Model file for the job. Use its own axes, mm. A direction names the side the tool comes from. Coordinates: 2 decimals unless noted, no trailing zeros. Loops run counter-clockwise (first coordinate to the right, second up) from the corner with the lowest first, then second, coordinate; pieces in that order, holes last.
from build123d import *

# Parameters (mm, degrees)
EXTRUDE_1_DEPTH        = 3.5
EXTRUDE_2_DEPTH        = 1.5
SKETCH_3_OUTSIDE_W     = 10.094
SKETCH_3_OUTSIDE_H     = 10.094
SKETCH_3_OUTSIDE_R     = 2.29
CUT_EXTRUDE_1_DEPTH    = 0.1
SKETCH_4_W             = 1
SKETCH_4_H             = 1.4
EXTRUDE_3_DEPTH        = 0.275
FILLET_1_R             = 0.1
FILLET_1_OF_MIRROR_1_R = 0.1
CUT_EXTRUDE_2_DEPTH    = 2


with BuildPart() as part:
    # 草图1 → 凸台-拉伸1 (new body)
    with BuildSketch(Plane.XY):
        Polygon((-1.91862915, -3.05), (1.91862915, -3.05), (3.05, -1.91862915), (3.05, 1.91862915), (1.91862915, 3.05), (-1.91862915, 3.05), (-3.05, 1.91862915), (-3.05, -1.91862915), align=None)
    extrude(amount=EXTRUDE_1_DEPTH)

    # 草图2 → 凸台-拉伸2 (add)
    with BuildSketch(Plane.XY.offset(3.5)):
        Polygon((2.29, -1.936446609), (1.936446609, -2.29), (-1.936446609, -2.29), (-2.29, -1.936446609), (-2.29, 1.936446609), (-1.936446609, 2.29), (1.936446609, 2.29), (2.29, 1.936446609), align=None)
    extrude(amount=EXTRUDE_2_DEPTH)

    # 草图3 outside → 切除-拉伸1 (cut)
    with BuildSketch(Plane.XY.offset(5)):
        Rectangle(SKETCH_3_OUTSIDE_W, SKETCH_3_OUTSIDE_H)
        Circle(SKETCH_3_OUTSIDE_R, mode=Mode.SUBTRACT)
    cut_extrude_1 = extrude(amount=-CUT_EXTRUDE_1_DEPTH, mode=Mode.SUBTRACT)

    # 草图4 → 凸台-拉伸3 (add)
    with BuildSketch(Plane.ZY.offset(3.05)):
        with Locations((0.5, 0)):
            Rectangle(SKETCH_4_W, SKETCH_4_H)
    extrude_3 = extrude(amount=EXTRUDE_3_DEPTH)

    # 圆角1
    fillet_1_edges = [part.edges().sort_by_distance(p)[0] for p in [
        (-3.325, 0, 1),
        (-3.325, 0, 0),
    ]]
    fillet(fillet_1_edges, radius=FILLET_1_R)

    # 镜向1: 切除-拉伸1, 凸台-拉伸3 across plane
    add(cut_extrude_1.mirror(Plane(origin=(0, 0, 0), x_dir=(0, 0, 1), z_dir=(1, 0, 0))), mode=Mode.SUBTRACT)
    add(extrude_3.mirror(Plane(origin=(0, 0, 0), x_dir=(0, 0, 1), z_dir=(1, 0, 0))))

    # 圆角1 of 镜向1
    fillet_1_of_mirror_1_edges = [part.edges().sort_by_distance(p)[0] for p in [
        (3.325, 0, 1),
        (3.325, 0, 0),
    ]]
    fillet(fillet_1_of_mirror_1_edges, radius=FILLET_1_OF_MIRROR_1_R)

    # 草图5 → 切除-拉伸2 (cut)
    with BuildSketch(Plane.XY.offset(3.5)):
        Polygon((-2.34, 1.936446609), (-2.34, -1.936446609), (-1.936446609, -2.34), (1.936446609, -2.34), (2.34, -1.936446609), (2.34, 1.936446609), (1.936446609, 2.328890946), (-1.936446609, 2.328890946), align=None)
        Polygon((-2.29, 1.936446609), (-1.936446609, 2.29), (1.936446609, 2.29), (2.29, 1.936446609), (2.29, -1.936446609), (1.936446609, -2.29), (-1.936446609, -2.29), (-2.29, -1.936446609), align=None, mode=Mode.SUBTRACT)
    extrude(amount=-CUT_EXTRUDE_2_DEPTH, mode=Mode.SUBTRACT)


solid = part.part
Q1. Flat gauge pins, fed straight in: P1, Ø1.7, axis at y = -0.5, z = 3, coming from the +X side; P2, Ø1, axis at x = -2.5, z = 1, coming from the -Y side; P3, Ø2.5, axis at y = -1, z = 4, coming from the -X side. Where does each tip first touch, or does it go through?
Answers:
P1: stops at x = 3.05
P2: stops at y = -2.97
P3: stops at x = -3.05
Q2. Which spindle directions (+Z, -Z, +X, -X, +Y, -Y) get a long thin tool onto all of the face, cutting with end or side? Do faces 1 (the flat face through (2, -2, 4.9)), 2 (the flat face through (0, -2.29, 4)), 3 (the flat face through (2, 2, 4.9)), 4 (the flat face through (0, 0, 0)). Say none if no direction does.
Answers:
face 1: +Z, +X, -Y
face 2: +Z
face 3: +Z, +X, +Y
face 4: -Z, +X, -X, +Y, -Y
Q3. Slice it at A-A (z = 3.1). List the corners of the cut face in (x, y).
Answers:
outline: (-3.05, -1.92) - (-1.92, -3.05) - (1.92, -3.05) - (3.05, -1.92) - (3.05, 1.92) - (1.92, 3.05) - (-1.92, 3.05) - (-3.05, 1.92) - close; (-2.29, -1.94) - (-1.94, -2.29) - (1.94, -2.29) - (2.29, -1.94) - (2.29, 1.94) - (1.94, 2.29) - (-1.94, 2.29) - (-2.29, 1.94) - close; hole (-2.34, -1.94) - (-1.94, -2.34) - (1.94, -2.34) - (2.34, -1.94) - (2.34, 1.94) - (1.94, 2.33) - (-1.94, 2.33) - (-2.34, 1.94) - close
Q4. Drill centre lines: line 1 (Z direction, x = 1.5, y = 2.75); line 2 (X direction, y = -1.75, z = 0.65); line 3 (Y direction, x = 1.5, z = 3.7). Where is each one in solid material? Low to high.
Answers:
line 1: z = 0 to 3.5
line 2: x = -3.05 to 3.05
line 3: y = -2.29 to 2.29
Q5. Slice it at D-D (y = -1.25). List the corners of the cut face in (x, z).
Answers:
outline: (-3.05, 0) - (3.05, 0) - (3.05, 3.5) - (2.34, 3.5) - (2.34, 1.5) - (2.29, 1.5) - (2.29, 4.9) - (1.92, 4.9) - (1.92, 5) - (-1.92, 5) - (-1.92, 4.9) - (-2.29, 4.9) - (-2.29, 1.5) - (-2.34, 1.5) - (-2.34, 3.5) - (-3.05, 3.5) - close
Q6. Mould opens along X. For faces 5 (the flat face through (0, 2.29, 4)), 6 (the flat face through (-2.49, -2.48, 1.73)), 7 (the flat face through (2.49, 2.48, 1.73)) say: +X half, -X half, draft (parallel to the pull), parting line (faces both ways), or undercut.
Answers:
face 5: undercut
face 6: -X half
face 7: +X half
Q7. Slice it at B-B (z = 1.15). List the corners of the cut face in (x, y), and give its area (4 significant figures).
Answers:
outline: (-3.05, -1.92) - (-1.92, -3.05) - (1.92, -3.05) - (3.05, -1.92) - (3.05, 1.92) - (1.92, 3.05) - (-1.92, 3.05) - (-3.05, 1.92) - close
area: 34.65 mm2
